Work out the finished part from the listing and answer in its coordinate system (mm). Face numbers are marked on the shaded views. A direction names the side the tool comes from. Round coordinates to 2 decimals unless told otherwise and drop trailing zeros. Loops run counter-clockwise (first coordinate to the right, second up) from the corner with the lowest first, then second, coordinate; pieces in that order, holes last.
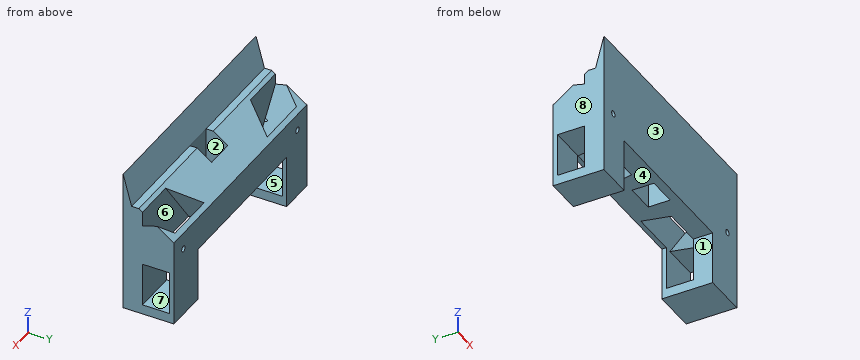
from build123d import *

# Parameters (mm, degrees)
BOSS_EXTRUDE2_DEPTH        = 25
SKETCH4_W                  = 18
SKETCH4_H                  = 11.172071032
CUT_EXTRUDE1_DEPTH         = 110.64235231
CUT_SWEEP3_START           = -47.833237702
CUT_SWEEP3_DEPTH           = 40.241500367
CUT_SWEEP4_START           = 2.134725454
CUT_SWEEP4_DEPTH           = 40.561080438
SKETCH24_W                 = 3
SKETCH24_H                 = 22.191771217
CUT_EXTRUDE15_DEPTH        = 15
CORTAR_EXTRUIR1_DEPTH      = 110.64235231
CORTAR_EXTRUIR1_DEPTH_BACK = 110.64235231
CORTAR_EXTRUIR2_DEPTH      = 110.64235231
CORTAR_EXTRUIR2_DEPTH_BACK = 110.64235231
CORTAR_EXTRUIR3_DEPTH      = 76.49647267
CORTAR_EXTRUIR3_DEPTH_BACK = 76.49647267
CORTAR_EXTRUIR4_DEPTH      = 108.627401408
CORTAR_EXTRUIR4_DEPTH_BACK = 108.627401408
CORTAR_EXTRUIR7_DEPTH      = 68.452835826
CORTAR_EXTRUIR7_DEPTH_BACK = 68.452835826
CROQUIS9_R                 = 1.245
CORTAR_EXTRUIR6_DEPTH      = 67.906302907
CORTAR_EXTRUIR6_DEPTH_BACK = 10


# Read off the part's stored shape, not the designer's step: Cut-Sweep3, Cut-Sweep4
with BuildPart() as part:
    # Sketch1 → Boss-Extrude2 (new body)
    with BuildSketch(Plane(origin=(0, 0, 0), x_dir=(1, 0, 0), z_dir=(0, 1, 0))):
        Polygon((26.674798416, 25.056972824), (44.674798416, 25.056972824), (44.674798416, -39.943027176), (-54.325201584, -39.943027176), (-54.325201584, 25.056972824), (-36.325201584, 25.056972824), (-36.325201584, 10.056972824), (26.674798416, 10.056972824), align=None)
    extrude(amount=BOSS_EXTRUDE2_DEPTH)

    # Sketch4 → Cut-Extrude1 (cut, through all)
    with BuildSketch(Plane(origin=(44.674798416, 0, 0), x_dir=(0, 0, -1), z_dir=(1, 0, 0))):
        Polygon((-39.943027176, 25), (-39.943027176, 0), (-21.024366767, 6.487240423), (-7.943027176, 25), align=None)
        with Locations((12.056972824, 13.586035516)):
            Rectangle(SKETCH4_W, SKETCH4_H)
    extrude(amount=-CUT_EXTRUDE1_DEPTH, mode=Mode.SUBTRACT)

    # Cut-Sweep3 outline → Cut-Sweep3 (cut)
    with BuildSketch(Plane(origin=(0, 0, 0), x_dir=(0.8133953590059209, 0, 0.5817112599457132), z_dir=(0.5817112599457132, 0, -0.8133953590059209)).offset(CUT_SWEEP3_START)):
        Polygon((-17.497304793, -8), (-35.180519898, -8), (-33.55372918, -19.172071032), (-15.870514075, -19.172071032), align=None)
    extrude(amount=CUT_SWEEP3_DEPTH, mode=Mode.SUBTRACT)

    # Cut-Sweep4 outline → Cut-Sweep4 (cut)
    with BuildSketch(Plane(origin=(0, 0, 0), x_dir=(0.8018445876826973, 0, -0.5975326411201026), z_dir=(0.5975326411201026, 0, 0.8018445876826972)).offset(CUT_SWEEP4_START)):
        Polygon((10.094047266, 8), (27.526148602, 8), (25.412737953, 19.172071032), (7.980636617, 19.172071032), align=None)
    extrude(amount=CUT_SWEEP4_DEPTH, mode=Mode.SUBTRACT)

    # Sketch24 → Cut-Extrude15 (cut)
    with BuildSketch(Plane(origin=(0, 0, -25.056972824), x_dir=(-1, 0, 0), z_dir=(0, 0, -1))):
        with Locations((37.825201584, 11.095885609)):
            Rectangle(SKETCH24_W, SKETCH24_H)
    extrude(amount=-CUT_EXTRUDE15_DEPTH, mode=Mode.SUBTRACT)

    # Croquis2 → Cortar-Extruir1 (cut, two sides: drawn at the far end of the back side and taken through both)
    with BuildSketch(Plane(origin=(44.674798416, 0, 0), x_dir=(0, 0, -1), z_dir=(1, 0, 0)).offset(-CORTAR_EXTRUIR1_DEPTH_BACK)):
        Polygon((-21.024366767, 5.069239779), (-21.024366767, 6.487240423), (-39.943027176, 0), align=None)
    extrude(amount=CORTAR_EXTRUIR1_DEPTH + CORTAR_EXTRUIR1_DEPTH_BACK, mode=Mode.SUBTRACT)

    # Croquis3 → Cortar-Extruir2 (cut, two sides: drawn at the far end of the back side and taken through both)
    with BuildSketch(Plane(origin=(44.674798416, 0, 0), x_dir=(0, 0, -1), z_dir=(1, 0, 0)).offset(-CORTAR_EXTRUIR2_DEPTH_BACK)):
        Polygon((-21.024366767, 3.483339502), (-21.024366767, 5.069239779), (-39.943027176, 0), (-34.024366767, 0), align=None)
    extrude(amount=CORTAR_EXTRUIR2_DEPTH + CORTAR_EXTRUIR2_DEPTH_BACK, mode=Mode.SUBTRACT)

    # Croquis4 → Cortar-Extruir3 (cut, two sides: drawn at the far end of the back side and taken through both)
    with BuildSketch(Plane.XY.offset(21.024366767).offset(-CORTAR_EXTRUIR3_DEPTH_BACK)):
        Polygon((-4.825201584, 3.483339502), (1.234798416, 3.483339502), (1.234798416, 12.513339502), (-4.795201584, 12.513339502), (-10.825201584, 12.513339502), (-10.825201584, 3.483339502), align=None)
    extrude(amount=CORTAR_EXTRUIR3_DEPTH + CORTAR_EXTRUIR3_DEPTH_BACK, mode=Mode.SUBTRACT)

    # Croquis5 → Cortar-Extruir4 (cut, two sides: drawn at the far end of the back side and taken through both)
    with BuildSketch(Plane(origin=(44.674798416, 0, 0), x_dir=(0, 0, -1), z_dir=(1, 0, 0)).offset(-CORTAR_EXTRUIR4_DEPTH_BACK)):
        Polygon((-10.769475505, 21), (-7.943027176, 21), (25.056972824, 21), (25.056972824, 25), (-7.943027176, 25), align=None)
    extrude(amount=CORTAR_EXTRUIR4_DEPTH + CORTAR_EXTRUIR4_DEPTH_BACK, mode=Mode.SUBTRACT)

    # Croquis9 → Cortar-Extruir7 (cut, two sides: drawn at the far end of the back side and taken through both)
    with BuildSketch(Plane(origin=(0, 21, 0), x_dir=(1, 0, 0), z_dir=(0, 1, 0)).offset(-CORTAR_EXTRUIR7_DEPTH_BACK)):
        with Locations(Location((-47.325201584, -3.856251341, 0), (0, 0, 270))):
            Circle(CROQUIS9_R)
        with Locations(Location((37.674798416, -3.856251341, 0), (0, 0, 270))):
            Circle(CROQUIS9_R)
    extrude(amount=CORTAR_EXTRUIR7_DEPTH + CORTAR_EXTRUIR7_DEPTH_BACK, mode=Mode.SUBTRACT)

    # Croquis7 → Cortar-Extruir6 (cut, two sides: drawn at the far end of the back side and taken through both)
    with BuildSketch(Plane.XZ.offset(-19.172071032).offset(-CORTAR_EXTRUIR6_DEPTH_BACK)):
        Polygon((-4.825201584, -3.056972824), (26.674798416, -3.056972824), (26.674798416, -10.056972824), (-4.825201584, -10.056972824), (-39.325201584, -10.056972824), (-39.325201584, -3.056972824), align=None)
    extrude(amount=CORTAR_EXTRUIR6_DEPTH + CORTAR_EXTRUIR6_DEPTH_BACK, mode=Mode.SUBTRACT)


solid = part.part
Item 1: Section A-A, the plane y = 11.5 is taken. Give the vertices of the cut face in (x, z) (3 decimals).
Item 2: Section C-C, the plane x = -30.5 is taken. Give the vertices of the cut face in (y, z), plus the area to 3 significant figures.
Item 3: For the marked faces 1, 2, 3, 4 and 5, determine the directions among +Z, -Z, +X, -X, +Y, -Y from which every point of the face is accessible in a straight line to the end or side of a thin tool.
Item 4: Section B-B, the plane z = -12.5 is taken. Give the vertices of the cut face in (x, y), plus the area to 3 significant figures.
Item 5: Section D-D, the plane y = 5 is taken. Give the vertices of the cut face in (x, z) (3 decimals).
Item 6: Determine the mould class of the marked faces 6, 7 and 8 for opening direction X: pulls with the +X half, pulls with the -X half, needs draft (parallel to the pull), parting line crosses it, or undercut.
Item 7: Straight lines are drawn through the part: line 1 (X direction, y = 1, z = -13); line 2 (X direction, y = 18.5, z = 6.5); line 3 (Y direction, x = 29.5, z = -5). For each, find the intervals that lie inside material, in ascending order.
Item 8: Each of these flat-tipped pins is pushed along its axis until it touches: P1, Ø5.5, axis at x = -46.5, y = 11.5, coming from the +Z side; P2, Ø4.5, axis at x = -38.5, z = 2, coming from the -Y side; P3, Ø9, axis at x = 37, y = 14, coming from the +Z side; P4, Ø3.5, axis at x = -35, y = 5.5, coming from the +Z side. Where does it stop, or does it pass through?
Answer below:
1. outline: (-54.325, -25.057) - (-39.325, -25.057) - (-39.325, -21.057) - (-54.325, -21.057) - close; (-54.325, -3.057) - (-40.439, -3.057) - (-54.325, 16.36) - close; (-33.388, 17.482) - (-18.699, -3.057) - (-10.825, -3.057) - (-10.825, 17.482) - close; (1.235, -3.057) - (9.485, -3.057) - (24.791, 17.482) - (1.235, 17.482) - close; (26.675, -25.057) - (44.675, -25.057) - (44.675, -21.057) - (26.675, -21.057) - close; (31.225, -3.057) - (44.675, -3.057) - (44.675, 14.992) - (37.248, 5.026) arc R1.245 cw (long way) to (36.432, 3.931) - close; hole circle Ø2.49 at (-47.325, 3.856)
2. outline: (0, -3.06) - (8, -3.06) - (8, 12.57) - (15.72, 14.5) - (6.49, 21.02) - (3.48, 21.02) - (0, 34.02) - close; (19.17, -3.06) - (21, -3.06) - (21, 10.77) - (19.17, 12.06) - close
2. area: 269 mm2
3. face 1: -Z, +Y, -Y
3. face 2: +Z, -Z
3. face 3: +Z, -Z, +X, -X, -Y
3. face 4: none
3. face 5: +X, -X
4. outline: (-54.33, 0) - (-39.33, 0) - (-39.33, 8) - (-54.33, 8) - close; (-54.33, 19.17) - (-39.33, 19.17) - (-39.33, 21) - (-54.33, 21) - close; (26.67, 0) - (44.67, 0) - (44.67, 8) - (26.67, 8) - close; (26.67, 19.17) - (44.67, 19.17) - (44.67, 21) - (26.67, 21) - close
4. area: 324 mm2
5. outline: (-54.325, -25.057) - (-39.325, -25.057) - (-39.325, -3.057) - (-10.825, -3.057) - (-10.825, 21.024) - (-54.325, 21.024) - close; (1.235, -3.057) - (26.675, -3.057) - (26.675, -25.057) - (44.675, -25.057) - (44.675, 21.024) - (1.235, 21.024) - close; hole circle Ø2.49 at (-47.325, 3.856); hole circle Ø2.49 at (37.675, 3.856)
6. face 6: undercut
6. face 7: needs draft
6. face 8: pulls with the -X half
7. line 1: x = -54.33 to -39.33, 26.67 to 44.67
7. line 2: x = -54.33 to -46.02, -24.28 to 14.96, 36.7 to 44.67
7. line 3: y = 0 to 8, 19.17 to 21
8. P1: stops at z = 9.32
8. P2: stops at y = 0
8. P3: stops at z = 11.69
8. P4: stops at z = 21.02
